Input: part model. Units: mm. Frame: model coordinates. Face numbers are marked on the shaded views. A direction names the side the tool comes from. Coordinates: 2 decimals unless noted, no trailing zeros. Write each loop counter-clockwise with the first axis right and the second up, starting at its lowest first coordinate (ties: lowest second). Pieces come first, ordered by that corner, then holes. Notation, with made-up numbers: M 69,25.25 L 96,25.25 A22 cw 96,49.25 Z; hole C 43.5,49.25 d5. An arc over 180 degrees is marked long. Answer as a JSON object with one key per item and string values. Group by question number.
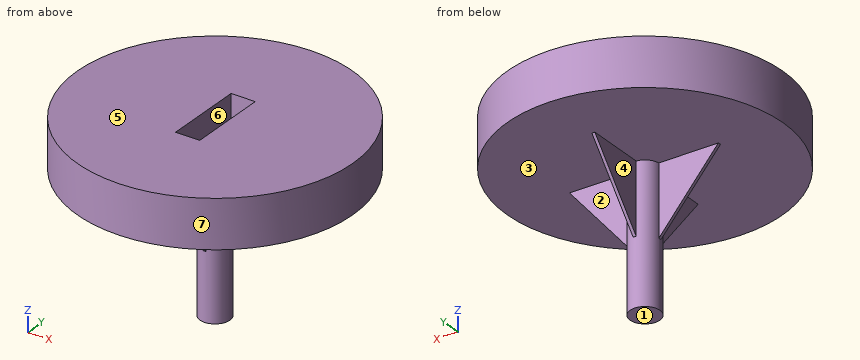
from build123d import *

# Parameters (mm, degrees)
CYLINDER_R                 = 4
CYLINDER_DEPTH             = 40
BOX002_W                   = 40
BOX002_H                   = 0.8
BOX002_DEPTH               = 20
CHAMFER_1_SIZE2            = 16
CHAMFER_1_SIZE             = 19
CHAMFER_2_SIZE2            = 16
CHAMFER_2_SIZE             = 19
BOX003_W                   = 40
BOX003_H                   = 0.8
BOX003_DEPTH               = 20
CHAMFER001_1_SIZE2         = 16
CHAMFER001_1_SIZE          = 19
CHAMFER001_2_SIZE2         = 16
CHAMFER001_2_SIZE          = 19
CHAMFER001_PLACEMENT_ANGLE = 90
BOX001_W                   = 6.5
BOX001_H                   = 21.5
BOX001_DEPTH               = 10
CYLINDER002_R              = 37
CYLINDER002_DEPTH          = 13


with BuildPart() as obj1:
    # Cylinder → Cylinder (new body)
    with BuildSketch(Plane.XY.offset(-10)):
        Circle(CYLINDER_R)
    extrude(amount=CYLINDER_DEPTH)


with BuildPart() as chamfer_body:
    # Box002 → Box002 (new body)
    with BuildSketch(Plane(origin=(-20, -0.4, 8), x_dir=(1, 0, 0), z_dir=(0, 0, 1))):
        with Locations((20, 0.4)):
            Rectangle(BOX002_W, BOX002_H)
    extrude(amount=BOX002_DEPTH)

    # Chamfer 1
    chamfer_1_edges = [chamfer_body.edges().sort_by_distance(p)[0] for p in [
        (20, 0, 8),
    ]]
    chamfer_1_side = chamfer_body.faces().sort_by_distance((20, 0, 18))[0]
    chamfer(chamfer_1_edges, length=CHAMFER_1_SIZE, length2=CHAMFER_1_SIZE2, reference=chamfer_1_side)

    # Chamfer 2
    chamfer_2_edges = [chamfer_body.edges().sort_by_distance(p)[0] for p in [
        (-20, 0, 8),
    ]]
    chamfer_2_side = chamfer_body.faces().sort_by_distance((-20, 0, 18))[0]
    chamfer(chamfer_2_edges, length=CHAMFER_2_SIZE, length2=CHAMFER_2_SIZE2, reference=chamfer_2_side)


with BuildPart() as chamfer001:
    # Box003 → Box003 (new body)
    with BuildSketch(Plane(origin=(-20, -0.4, 8), x_dir=(1, 0, 0), z_dir=(0, 0, 1))):
        with Locations((20, 0.4)):
            Rectangle(BOX003_W, BOX003_H)
    extrude(amount=BOX003_DEPTH)

    # Chamfer001 1
    chamfer001_1_edges = [chamfer001.edges().sort_by_distance(p)[0] for p in [
        (20, 0, 8),
    ]]
    chamfer001_1_side = chamfer001.faces().sort_by_distance((20, 0, 18))[0]
    chamfer(chamfer001_1_edges, length=CHAMFER001_1_SIZE, length2=CHAMFER001_1_SIZE2, reference=chamfer001_1_side)

    # Chamfer001 2
    chamfer001_2_edges = [chamfer001.edges().sort_by_distance(p)[0] for p in [
        (-20, 0, 8),
    ]]
    chamfer001_2_side = chamfer001.faces().sort_by_distance((-20, 0, 18))[0]
    chamfer(chamfer001_2_edges, length=CHAMFER001_2_SIZE, length2=CHAMFER001_2_SIZE2, reference=chamfer001_2_side)


with BuildPart() as chamfer001_1:
    # Chamfer001 placement: moved
    add(chamfer001.part.rotate(Axis((0, 0, 0), (0, 0, 1)), CHAMFER001_PLACEMENT_ANGLE))


with BuildPart() as obj2:
    # Box001 → Box001 (new body)
    with BuildSketch(Plane(origin=(-3.25, -10.6, 30), x_dir=(1, 0, 0), z_dir=(0, 0, 1))):
        with Locations((3.25, 10.75)):
            Rectangle(BOX001_W, BOX001_H)
    extrude(amount=BOX001_DEPTH)


with BuildPart() as obj3:
    # Cylinder002 → Cylinder002 (new body)
    with BuildSketch(Plane.XY.offset(27)):
        Circle(CYLINDER002_R)
    extrude(amount=CYLINDER002_DEPTH)

    # Cut: cut obj2
    add(obj2.part, mode=Mode.SUBTRACT)

    # Fusion: union obj1, Chamfer body, Chamfer001
    add(obj1.part)
    add(chamfer_body.part)
    add(chamfer001_1.part)


solid = obj3.part
Q1. Section D-D, the plane x = -26. Return the cut outline in (y, z).
Q2. Section A-A, the plane z = 34.5. Return the cut outline in (x, y).
Q3. Line query: line 1 (Y direction, x = 1, z = 31.5); line 2 (Z direction, x = -10.5, y = -8.5); line 3 (Y direction, x = 6.5, z = 16). Output: solid intervals per line, ascending. Write a range as from..to.
Q4. Access query for the marked faces 1, 2, 3 and 4. Directions: +Z, -Z, +X, -X, +Y, -Y. A direction counts if a zero-diameter tool reaches every point of the face in a straight line with its end or side. Return the directions, or none.
Q5. Pin query (flat end, axial travel): pin 1 Ø17.5 at (y, z) = (-12, 15.5) entering from +X; pin 2 Ø5 at (x, z) = (1, 35) entering from -Y; pin 3 Ø2 at (x, z) = (-1.5, 36.5) entering from +Y; pin 4 Ø1 at (y, z) = (-26.5, 25.5) entering from -X. Return the tip coordinate at first contact, or that it passes through.
Q6. Draft query along X for the marked faces 5, 6 and 7. Return one class per face: released by +X, released by -X, zero draft, split by the parting line, or undercut.
Q7. Section C-C, the plane z = 22. Return the cut outline in (x, y).
Q8. Section B-B, the plane y = 2. Return the cut outline in (x, z), and give its area (3 significant figures).
Filled in:
{
 "1": {"outline": "M -26.32,27 L 26.32,27 L 26.32,40 L -26.32,40 Z"},
 "2": {"outline": "C 0,0 d74; hole M -3.25,-10.6 L 3.25,-10.6 L 3.25,10.9 L -3.25,10.9 Z"},
 "3": {"line 1": "-36.99..-10.6, 10.9..36.99", "line 2": "27..40", "line 3": "-0.4..0.4"},
 "4": {"face 1": "-Z, +X, -X, +Y, -Y", "face 2": "-Z, +X, +Y", "face 3": "-Z", "face 4": "-Z, -X, +Y"},
 "5": {"pin 1": "x = 2.33", "pin 2": "y = -37", "pin 3": "y = 37", "pin 4": "through"},
 "6": {"face 5": "zero draft", "face 6": "undercut", "face 7": "split by the parting line"},
 "7": {"outline": "M -15.79,-0.4 L -3.98,-0.4 A4 ccw -0.4,-3.98 L -0.4,-15.79 L 0.4,-15.79 L 0.4,-3.98 A4 ccw 3.98,-0.4 L 15.79,-0.4 L 15.79,0.4 L 3.98,0.4 A4 ccw 0.4,3.98 L 0.4,15.79 L -0.4,15.79 L -0.4,3.98 A4 ccw -3.98,0.4 L -15.79,0.4 Z"},
 "8": {"outline": "M -36.95,27 L -3.46,27 L -3.46,-10 L 3.46,-10 L 3.46,27 L 36.95,27 L 36.95,40 L 3.25,40 L 3.25,30 L -3.25,30 L -3.25,40 L -36.95,40 Z", "area": "1,150 mm^2"}
}
